Can you work these out from the model? Positions are in its coordinate system, mm. Face numbers are marked on the shaded views. Give positions to 0.01 mm unless a question says otherwise; leave off trailing zeros. Order: outer loops, then holes, each group sorted by start corner. A loop starts at its lowest first (then second) coordinate and runs counter-clockwise, first axis right, second up. Notation, with made-up numbers: (-19, -7.75) - (25, -7.75) arc R32 ccw to (25, 28.25) - close; hole circle Ø5 at (15.5, -9.5). An arc over 180 degrees is marked (long way). Answer as a JSON object with one key per item and string values.
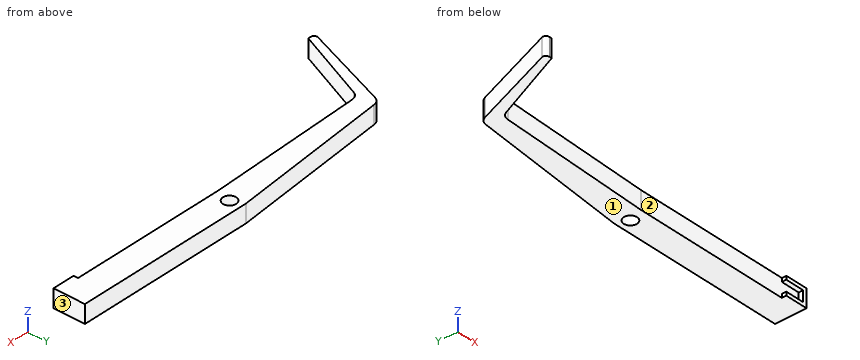
```python
from build123d import *

# Parameters (mm, degrees)
BOSS_EXTRUDE1_DEPTH     = 8
SKETCH6_W               = 1.6
SKETCH6_H               = 2.4
BOSS_EXTRUDE2_DEPTH     = 2
FILLET1_R               = 4
CUT_EXTRUDE1_DEPTH      = 101.380345151
CUT_EXTRUDE1_DEPTH_BACK = 101.380345151
SKETCH7_R               = 2.966503931
FILLET3_R               = 1.5


with BuildPart() as part:
    # Sketch4 → Boss-Extrude1 (new body)
    with BuildSketch(Plane.XY):
        Polygon((77.746809309, 38.75), (-2.253190691, 38.75), (-76.855180537, 31.033581723), (-92.253190691, -11.25), (-88.923190691, -11.25), (-74.253190691, 23.75), (-2.253190691, 26.75), (77.746809309, 26.75), align=None)
    extrude(amount=BOSS_EXTRUDE1_DEPTH)

    # Sketch6 → Boss-Extrude2 (add)
    with BuildSketch(Plane.XZ.offset(-26.75)):
        Polygon((77.746809309, 6.4), (77.746809309, 8), (67.746809309, 8), (67.746809309, 6.4), (76.146809309, 6.4), align=None)
        with Locations((76.946809309, 5.2)):
            Rectangle(SKETCH6_W, SKETCH6_H)
        with Locations((76.946809309, 2.8)):
            Rectangle(SKETCH6_W, SKETCH6_H)
        Polygon((77.746809309, 0), (77.746809309, 1.6), (76.146809309, 1.6), (67.746809309, 1.6), (67.746809309, 0), align=None)
    extrude(amount=BOSS_EXTRUDE2_DEPTH)

    # Fillet1
    fillet1_edges = [part.edges().sort_by_distance(p)[0] for p in [
        (-74.253190691, 23.75, 4),
        (-76.855180537, 31.033581723, 4),
    ]]
    fillet(fillet1_edges, radius=FILLET1_R)

    # Sketch7 → Cut-Extrude1 (cut, two sides: drawn at the far end of the back side and taken through both)
    with BuildSketch(Plane.XY.offset(8).offset(-CUT_EXTRUDE1_DEPTH_BACK)):
        with Locations((0, 33.532902176)):
            Circle(SKETCH7_R)
    extrude(amount=CUT_EXTRUDE1_DEPTH + CUT_EXTRUDE1_DEPTH_BACK, mode=Mode.SUBTRACT)

    # Fillet3
    fillet3_edges = [part.edges().sort_by_distance(p)[0] for p in [
        (-92.253190691, -11.25, 4),
    ]]
    fillet(fillet3_edges, radius=FILLET3_R)


solid = part.part
```
Q1. If we section it at D-D, the plane y = -1.5: Please give me the cut outline in (x, z), then the cut area to 3 significant figures.
Recorded:
{"outline": "(-88.7, 0) - (-84.84, 0) - (-84.84, 8) - (-88.7, 8) - close", "area": "30.9 mm^2"}
Q2. I'm going to push flat-ended pins straight in: pin 1 Ø0.5 at (y, z) = (25.5, 7) entering from -X; pin 2 Ø1.5 at (y, z) = (25, 3) entering from -X; pin 3 Ø1.5 at (y, z) = (3.5, 5) entering from -X; pin 4 Ø10 at (x, y) = (-60, 16.5) entering from +Z. Where does each tip first touch, or does it pass through?
Recorded:
{"pin 1": "stops at x = -78.96", "pin 2": "stops at x = -79.33", "pin 3": "stops at x = -87.15", "pin 4": "passes through"}
Q3. We'd pull the mould along X, two halves only. Please class the marked faces 1, 2 and 3: released by +X, released by -X, zero draft, split by the parting line, or undercut.
Recorded:
{"face 1": "zero draft", "face 2": "undercut", "face 3": "released by +X"}
Q4. If we section it at C-C, the plane x = 24: Please give me the cut outline in (y, z), then the cut area to 3 significant figures.
Recorded:
{"outline": "(26.75, 0) - (38.75, 0) - (38.75, 8) - (26.75, 8) - close", "area": "96.0 mm^2"}
Q5. I need wall thicknesses on L1, parallel to Y at x = 0, z = 5.5; L2, parallel to Y at x = 51, z = 4.75; L3, parallel to Y at x = 68.5, z = 7.75. Which ranges of each line are inside material? Lowest first, please.
Recorded:
{"L1": "y = 26.75 to 30.57, 36.5 to 38.75", "L2": "y = 26.75 to 38.75", "L3": "y = 24.75 to 38.75"}
Q6. If we section it at B-B, the plane z = 5: Please give me the cut outline in (x, y), then the cut area to 3 significant figures.
Recorded:
{"outline": "(-91.52, -9.24) arc R1.5 ccw to (-90.11, -11.25) - (-88.92, -11.25) - (-75.24, 21.41) arc R4 cw to (-71.71, 23.86) - (-2.25, 26.75) - (76.15, 26.75) - (76.15, 24.75) - (77.75, 24.75) - (77.75, 38.75) - (-2.25, 38.75) - (-74.36, 31.29) arc R4 ccw to (-77.71, 28.68) - close; hole circle Ø5.93 at (0, 33.53)", "area": "1,820 mm^2"}
Q7. If we section it at A-A, the plane x = 0: Please give me the cut outline in (y, z).
Recorded:
{"outline": "(26.75, 0) - (30.57, 0) - (30.57, 8) - (26.75, 8) - close; (36.5, 0) - (38.75, 0) - (38.75, 8) - (36.5, 8) - close"}
